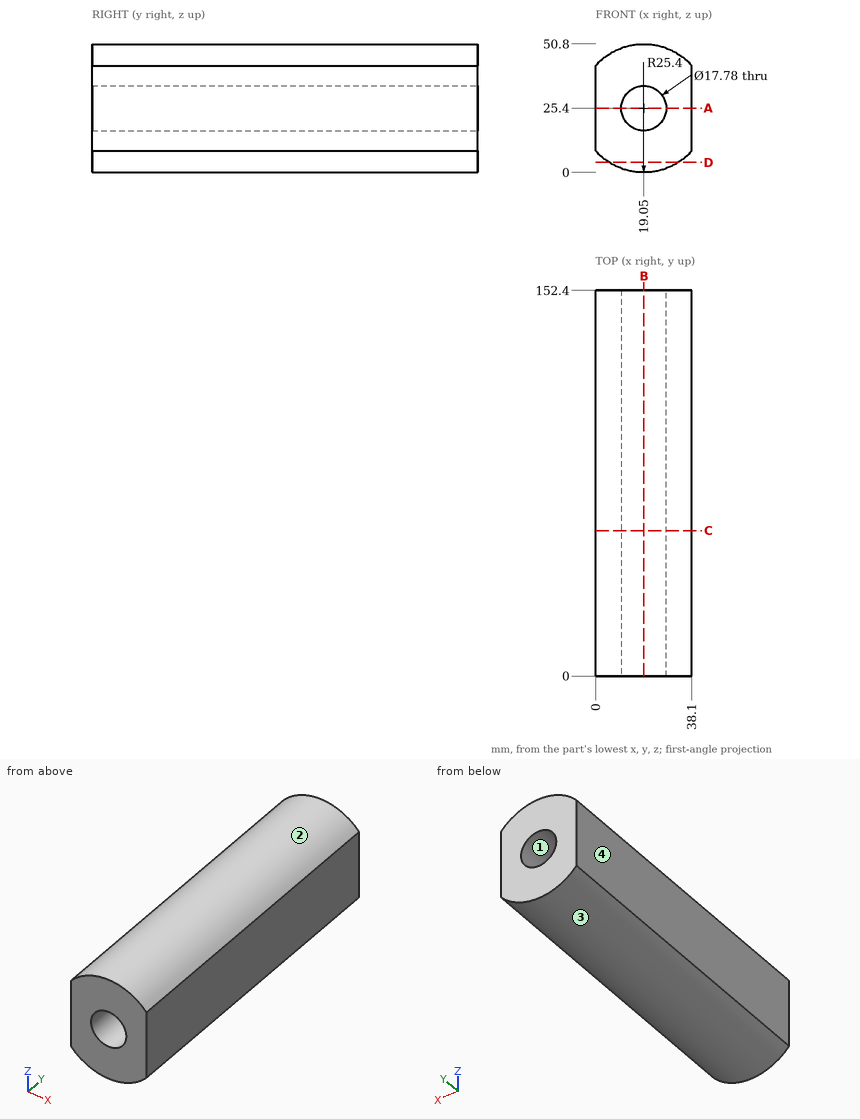
Input: dimensioned drawing with shaded views. Units: mm. Origin: part minimum x, y, z. Give positions to 0.01 mm unless a question says otherwise; leave off trailing zeros. Order: outer loops, then holes, each group sorted by start corner. A loop starts at its lowest first (then second) coordinate and runs counter-clockwise, first axis right, second up.
(1) Material intervals for line 1 along Z through (x, y) = (19.05, 87); line 2 along X through (y, z) = (91, 25.4); line 3 along Z through (x, y) = (15.5, 126.5), sorted ascending.
(2) Section query D-D (z = 4). Return the cut outline in (x, y), plus the area to 3 significant figures.
(3) Pull-direction query (Z, two-part tool) for the marked faces 1, 2, 3 and 4; classes: +Z half, -Z half, draft (parallel to the pull), parting line (faces both ways), or undercut.
(4) Section query B-B (x = 19.05). Return the cut outline in (y, z).
(5) Section query A-A (z = 25.4). Return the cut outline in (x, y).
(6) Section query C-C (y = 57.5). Return the cut outline in (x, z).
(7) Contact query for flat-ended pins moving along their axis: P1, Ø4, axis at x = 26.5, y = 131.5, coming from the +Z side; P2, Ø1.5, axis at x = 19.5, y = 58.5, coming from the +Z side; P3, Ø1, axis at x = 31, y = 63.5, coming from the +Z side. Output: stop coordinate, or through.
Outcome:
1. line 1: z = 0 to 16.51, 34.29 to 50.8
1. line 2: x = 0 to 10.16, 27.94 to 38.1
1. line 3: z = 0.25 to 17.25, 33.55 to 50.55
2. outline: (5.37, 0) - (32.73, 0) - (32.73, 152.4) - (5.37, 152.4) - close
2. area: 4,170 mm2
3. face 1: undercut
3. face 2: +Z half
3. face 3: -Z half
3. face 4: draft
4. outline: (0, 0) - (152.4, 0) - (152.4, 16.51) - (0, 16.51) - close; (0, 34.29) - (152.4, 34.29) - (152.4, 50.8) - (0, 50.8) - close
5. outline: (0, 0) - (10.16, 0) - (10.16, 152.4) - (0, 152.4) - close; (27.94, 0) - (38.1, 0) - (38.1, 152.4) - (27.94, 152.4) - close
6. outline: (0, 8.6) arc R25.4 ccw to (38.1, 8.6) - (38.1, 42.2) arc R25.4 ccw to (0, 42.2) - close; hole circle Ø17.78 at (19.05, 25.4)
7. P1: stops at z = 50.21
7. P2: stops at z = 50.8
7. P3: stops at z = 48.07
